Here's the drawing with two shaded views (mm, measured from the low corner). I have some questions. Give positions to 0.01 mm unless a question says otherwise; leave off trailing zeros. Order: outer loops, then holes, each group sorted by start corner. A loop starts at its lowest first (then second) coordinate and runs counter-clockwise, first axis right, second up. Notation, with made-up numbers: M 14,38 L 22,38 A23 ccw 22,53 Z; hole C 40,-18 d8. An arc over 180 degrees is marked long. Use a Markdown table: item, result. Add a question column.
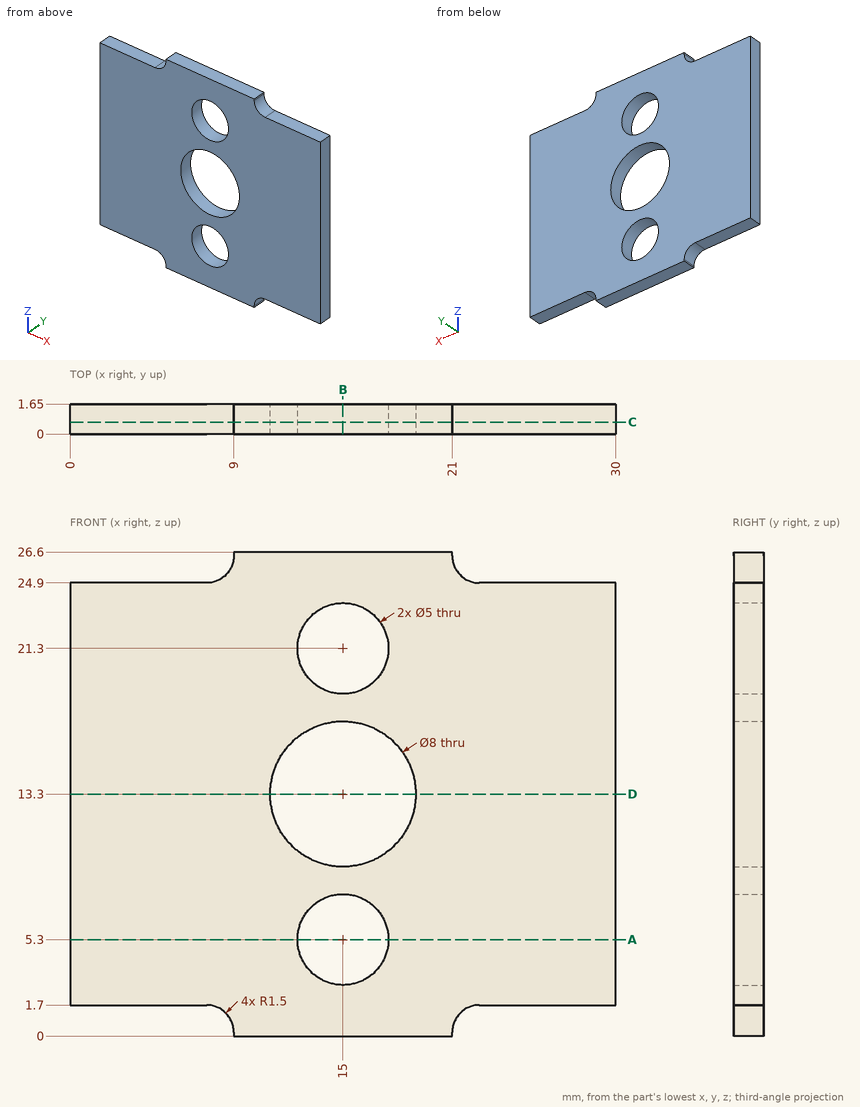
1. I need wall thicknesses on L1, parallel to Z at x = 15, y = 1.3; L2, parallel to Z at x = 14, y = 0.1; L3, parallel to X at y = 0.6, z = 21.3. Which ranges of each line are inside material? Lowest first, please. Write a range as [from, to].
2. If we section it at C-C, the plane y = 0.65: List the corners of the cut face in (x, z) for me, then the cut area to 3 significant figures.
3. Will these pins go through, and if not, where does the flat tip stop? pin 1 (5 mm diameter, centred on x = 24.5, z = 12, fed in from -Y); pin 2 (0.8 mm diameter, centred on x = 27, y = 0.5, fed in from -Z); pin 3 (0.5 mm diameter, centred on x = 28, y = 1, fed in from +Z).
4. If we section it at D-D, the plane z = 13.3: List the corners of the cut face in (x, y) for me, then the cut area to 3 significant figures.
5. If we section it at B-B, the plane x = 15: List the corners of the cut face in (y, z) for me, then the cut area to 3 significant figures.
6. If we section it at A-A, the plane z = 5.3: List the corners of the cut face in (x, y) for me.
Geometry results:
| question | item | result |
|---|---|---|
| 1 | L1 | z = [0, 2.8], [7.8, 9.3], [17.3, 18.8], [23.8, 26.6] |
| 1 | L2 | z = [0, 3.01], [7.59, 9.43], [17.17, 19.01], [23.59, 26.6] |
| 1 | L3 | x = [0, 12.5], [17.5, 30] |
| 2 | outline | M 0,1.7 L 7.5,1.7 A1.5 cw 9,0.2 L 9,0 L 21,0 L 21,0.2 A1.5 cw 22.5,1.7 L 30,1.7 L 30,24.9 L 22.5,24.9 A1.5 cw 21,26.4 L 21,26.6 L 9,26.6 L 9,26.4 A1.5 cw 7.5,24.9 L 0,24.9 Z; hole C 15,13.3 d8; hole C 15,5.3 d5; hole C 15,21.3 d5 |
| 2 | area | 649 mm^2 |
| 3 | pin 1 | stops at y = 0 |
| 3 | pin 2 | stops at z = 1.7 |
| 3 | pin 3 | stops at z = 24.9 |
| 4 | outline | M 0,0 L 11,0 L 11,1.65 L 0,1.65 Z; M 19,0 L 30,0 L 30,1.65 L 19,1.65 Z |
| 4 | area | 36.3 mm^2 |
| 5 | outline | M 0,0 L 1.65,0 L 1.65,2.8 L 0,2.8 Z; M 0,7.8 L 1.65,7.8 L 1.65,9.3 L 0,9.3 Z; M 0,17.3 L 1.65,17.3 L 1.65,18.8 L 0,18.8 Z; M 0,23.8 L 1.65,23.8 L 1.65,26.6 L 0,26.6 Z |
| 5 | area | 14.2 mm^2 |
| 6 | outline | M 0,0 L 12.5,0 L 12.5,1.65 L 0,1.65 Z; M 17.5,0 L 30,0 L 30,1.65 L 17.5,1.65 Z |
